from build123d import *

# Parameters (mm, degrees)
SKETCH1_W            = 39
SKETCH1_H            = 122
BOSS_EXTRUDE2_DEPTH  = 2
SKETCH2_W            = 2
SKETCH2_H            = 122
BOSS_EXTRUDE3_DEPTH  = 25
SKETCH3_W            = 2
SKETCH3_H            = 122
BOSS_EXTRUDE4_DEPTH  = 25
SKETCH4_W            = 35
SKETCH4_H            = 2
BOSS_EXTRUDE5_DEPTH  = 25
FILLET2_R            = 2
BOSS_EXTRUDE7_DEPTH  = 4
CUT_EXTRUDE2_DEPTH   = 4
SKETCH5_W            = 4
SKETCH5_H            = 9
CUT_EXTRUDE3_DEPTH   = 4
FILLET4_R            = 2
SKETCH8_W            = 7
SKETCH8_H            = 7
BOSS_EXTRUDE8_DEPTH  = 7
SKETCH9_W            = 7
SKETCH9_H            = 7
BOSS_EXTRUDE10_DEPTH = 7
SKETCH10_R           = 2
CUT_EXTRUDE6_DEPTH   = 7
SKETCH11_W           = 7
SKETCH11_H           = 7
BOSS_EXTRUDE11_DEPTH = 7
SKETCH12_R           = 2
CUT_EXTRUDE7_DEPTH   = 7


with BuildPart() as part:
    # Sketch1 → Boss-Extrude2 (new body)
    with BuildSketch(Plane.XY):
        with Locations((19.5, 61)):
            Rectangle(SKETCH1_W, SKETCH1_H)
    extrude(amount=BOSS_EXTRUDE2_DEPTH)

    # Sketch2 → Boss-Extrude3 (add)
    with BuildSketch(Plane(origin=(0, 0, 0), x_dir=(-1, 0, 0), z_dir=(0, 0, -1))):
        with Locations((-38, 61)):
            Rectangle(SKETCH2_W, SKETCH2_H)
    extrude(amount=BOSS_EXTRUDE3_DEPTH)

    # Sketch3 → Boss-Extrude4 (add)
    with BuildSketch(Plane(origin=(0, 0, 0), x_dir=(-1, 0, 0), z_dir=(0, 0, -1))):
        with Locations((-1, 61)):
            Rectangle(SKETCH3_W, SKETCH3_H)
    extrude(amount=BOSS_EXTRUDE4_DEPTH)

    # Sketch4 → Boss-Extrude5 (add)
    with BuildSketch(Plane(origin=(0, 0, 0), x_dir=(-1, 0, 0), z_dir=(0, 0, -1))):
        with Locations((-19.5, 1)):
            Rectangle(SKETCH4_W, SKETCH4_H)
    extrude(amount=BOSS_EXTRUDE5_DEPTH)

    # Fillet2
    fillet2_edges = [part.edges().sort_by_distance(p)[0] for p in [
        (19.5, 0, 2),
        (0, 0, -11.5),
        (39, 0, -11.5),
    ]]
    fillet(fillet2_edges, radius=FILLET2_R)

    # Sketch6 → Boss-Extrude7 (add)
    with BuildSketch(Plane(origin=(0, 0, -25), x_dir=(-1, 0, 0), z_dir=(0, 0, -1))):
        with BuildLine():
            Line((-2, 122), (0, 122))
            Line((0, 122), (0, 2))
            ThreePointArc((0, 2), (-0.585786438, 0.585786438), (-2, 0))
            Line((-2, 0), (-37, 0))
            ThreePointArc((-37, 0), (-38.414213562, 0.585786438), (-39, 2))
            Line((-39, 2), (-39, 122))
            Line((-39, 122), (-37, 122))
            Line((-37, 122), (-37, 2))
            Line((-37, 2), (-2, 2))
            Line((-2, 2), (-2, 122))
        make_face()
    extrude(amount=BOSS_EXTRUDE7_DEPTH)

    # Sketch7 → Cut-Extrude2 (cut)
    with BuildSketch(Plane.ZY):
        with BuildLine():
            Line((-21.5, 110), (-20.5, 110))
            ThreePointArc((-20.5, 110), (-19.439339828, 109.560660172), (-19, 108.5))
            Line((-19, 108.5), (-19, 102.5))
            ThreePointArc((-19, 102.5), (-19.439339828, 101.439339828), (-20.5, 101))
            Line((-20.5, 101), (-21.5, 101))
            ThreePointArc((-21.5, 101), (-22.560660172, 101.439339828), (-23, 102.5))
            Line((-23, 102.5), (-23, 108.5))
            ThreePointArc((-23, 108.5), (-22.560660172, 109.560660172), (-21.5, 110))
        make_face()
    extrude(amount=-CUT_EXTRUDE2_DEPTH, mode=Mode.SUBTRACT)

    # Sketch5 → Cut-Extrude3 (cut)
    with BuildSketch(Plane(origin=(39, 0, 0), x_dir=(0, 0, -1), z_dir=(1, 0, 0))):
        with Locations((21, 105.5)):
            Rectangle(SKETCH5_W, SKETCH5_H)
    extrude(amount=-CUT_EXTRUDE3_DEPTH, mode=Mode.SUBTRACT)

    # Fillet4
    # the kernel refuses this fillet: 2 mm, written as the material it takes off along each edge
    with BuildSketch(Plane(origin=(37, 2, 0), x_dir=(1, 0, 0), z_dir=(0, 0, 1))) as fillet4_piece_1_section:
        Polygon((0, 0), (FILLET4_R, 0), (FILLET4_R, -FILLET4_R), (0, -FILLET4_R), align=None)
    fillet4_piece_1 = extrude(amount=FILLET4_R, mode=Mode.PRIVATE)
    fillet4_piece_1 = fillet4_piece_1 - Plane(origin=(37, 2, 0), x_dir=(-0.7071067811865476, 0.7071067811865475, 0), z_dir=(0, 0, 1)) * Sphere(FILLET4_R, mode=Mode.PRIVATE)
    add(fillet4_piece_1, mode=Mode.SUBTRACT)
    with BuildSketch(Plane(origin=(2, 2, 0), x_dir=(0, 0, 1), z_dir=(-1, 0, 0))) as fillet4_piece_2_section:
        Polygon((0, 0), (FILLET4_R, 0), (FILLET4_R, -FILLET4_R), (0, -FILLET4_R), align=None)
    fillet4_piece_2 = extrude(amount=FILLET4_R, mode=Mode.PRIVATE)
    fillet4_piece_2 = fillet4_piece_2 - Plane(origin=(2, 2, 0), x_dir=(0, 0.7071067811865475, -0.7071067811865475), z_dir=(-1, 0, 0)) * Sphere(FILLET4_R, mode=Mode.PRIVATE)
    add(fillet4_piece_2, mode=Mode.SUBTRACT)
    with BuildSketch(Plane(origin=(0, 2, 2), x_dir=(0, 0, -1), z_dir=(0, 1, 0))) as fillet4_piece_3:
        with BuildLine():
            CenterArc((FILLET4_R, -FILLET4_R), FILLET4_R, 90, 90)
            Line((0, -FILLET4_R), (0, 0))
            Line((0, 0), (FILLET4_R, 0))
        make_face()
    extrude(amount=125, mode=Mode.SUBTRACT)
    with BuildSketch(Plane(origin=(39, 127, 2), x_dir=(-1, 0, 0), z_dir=(0, -1, 0))) as fillet4_piece_4:
        with BuildLine():
            CenterArc((FILLET4_R, FILLET4_R), FILLET4_R, 180, 90)
            Line((0, FILLET4_R), (0, 0))
            Line((0, 0), (FILLET4_R, 0))
        make_face()
    extrude(amount=125, mode=Mode.SUBTRACT)

    # Sketch8 → Boss-Extrude8 (add)
    with BuildSketch(Plane(origin=(0, 0, -29), x_dir=(-1, 0, 0), z_dir=(0, 0, -1))):
        with Locations((-33.5, 5.5)):
            Rectangle(SKETCH8_W, SKETCH8_H)
    extrude(amount=-BOSS_EXTRUDE8_DEPTH)

    # Sketch9 → Boss-Extrude10 (add)
    with BuildSketch(Plane(origin=(0, 0, -29), x_dir=(-1, 0, 0), z_dir=(0, 0, -1))):
        with Locations((-5.5, 5.5)):
            Rectangle(SKETCH9_W, SKETCH9_H)
    extrude(amount=-BOSS_EXTRUDE10_DEPTH)

    # Sketch10 → Cut-Extrude6 (cut)
    with BuildSketch(Plane(origin=(0, 0, -29), x_dir=(-1, 0, 0), z_dir=(0, 0, -1))):
        with Locations((-33.5, 5.5)):
            Circle(SKETCH10_R)
        with Locations((-5.5, 5.5)):
            Circle(SKETCH10_R)
    extrude(amount=-CUT_EXTRUDE6_DEPTH, mode=Mode.SUBTRACT)

    # Sketch11 → Boss-Extrude11 (add)
    with BuildSketch(Plane(origin=(0, 122, 0), x_dir=(1, 0, 0), z_dir=(0, 1, 0))):
        with Locations((5.5, 3.5)):
            Rectangle(SKETCH11_W, SKETCH11_H)
        with Locations((33.5, 3.5)):
            Rectangle(SKETCH11_W, SKETCH11_H)
        with Locations((5.5, 25.5)):
            Rectangle(SKETCH11_W, SKETCH11_H)
        with Locations((33.5, 25.5)):
            Rectangle(SKETCH11_W, SKETCH11_H)
    extrude(amount=-BOSS_EXTRUDE11_DEPTH)

    # Sketch12 → Cut-Extrude7 (cut)
    with BuildSketch(Plane(origin=(0, 122, 0), x_dir=(1, 0, 0), z_dir=(0, 1, 0))):
        with Locations(Location((5.5, 25.5, 0), (0, 0, 270))):
            Circle(SKETCH12_R)
        with Locations(Location((33.5, 25.5, 0), (0, 0, 270))):
            Circle(SKETCH12_R)
        with Locations(Location((5.5, 3.5, 0), (0, 0, 270))):
            Circle(SKETCH12_R)
        with Locations(Location((33.5, 3.5, 0), (0, 0, 270))):
            Circle(SKETCH12_R)
    extrude(amount=-CUT_EXTRUDE7_DEPTH, mode=Mode.SUBTRACT)


solid = part.part
Verification items for the finished model (mm, model axes). A direction names the side the tool comes from. Coordinates: 2 decimals unless noted, no trailing zeros. Write each loop counter-clockwise with the first axis right and the second up, starting at its lowest first coordinate (ties: lowest second). Pieces come first, ordered by that corner, then holes. Notation, with made-up numbers: (1.5, -30) -> (43.5, -30) arc R18 ccw to (43.5, -7) -> close; hole circle Ø3 at (37, 77). An arc over 180 degrees is marked (long way). One line per item, written item: value. Start each with the question number.
Q1. Go/stop test with a flat-tipped pin: P1, Ø4, axis at x = 12.5, z = -3.5, coming from the +Y side. Record where the tip stops, or that it passes through.
Q2. Cross-section at D-D on y = 5.5. Enter the section's corners in (x, z).
Q3. Access from +Z, -Z, +X, -X, +Y, -Y to the whole of each face (thin tool, end or side, straight path). Record for faces 5 (the flat face through (5, 119, -7)), 6 (the flat face through (34, 9, -26)), 7 (the flat face through (9, 119, -25)), 8 (the flat face through (1, 106, -19)).
Q4. Cross-section at C-C on x = 33.5. Enter the section's corners in (y, z).
Q5. Cross-section at A-A on z = -25.5. Enter the section's corners in (x, y), and give its area (3 significant figures).
Q6. Cross-section at B-B on z = -3.5. Enter the section's corners in (x, y), and give its area (3 significant figures).
Q7. Thickness scan on L1, parallel to X at y = 119.25, z = -3.5; L2, parallel to X at y = 5.5, z = -8.5; L3, parallel to X at y = 117, z = -25. Record the ranges inside material, lowest first. Write a range as from..to.
Q8. Mould release check, pull along X, two halves, no side actions. Record for faces 1 (the flat face through (39, 61, -14)), 2 (the flat face through (31.9, 115, -24)), 3 (the cylindrical face through (0.57, 61.16, 1.4)), 4 (the flat face through (30, 119, -25)): pulls with the +X half, pulls with the -X half, needs draft (parallel to the pull), parting line crosses it, or undercut.
Checked values:
1. P1: stops at y = 2
2. outline: (0, -29) -> (3.5, -29) -> (3.5, -22) -> (2, -22) -> (2, 0) -> (37, 0) -> (37, -22) -> (35.5, -22) -> (35.5, -29) -> (39, -29) -> (39, 0) arc R2 ccw to (37, 2) -> (2, 2) arc R2 ccw to (0, 0) -> close; (7.5, -29) -> (9, -29) -> (9, -22) -> (7.5, -22) -> close; (30, -29) -> (31.5, -29) -> (31.5, -22) -> (30, -22) -> close
3. face 5: +Y
3. face 6: -Z
3. face 7: -Z, +Y
3. face 8: +X, -X
4. outline: (0, -29) -> (3.5, -29) -> (3.5, -22) -> (2, -22) -> (2, 0) -> (115, 0) -> (115, -1.5) -> (122, -1.5) -> (122, 2) -> (2, 2) arc R2 ccw to (0, 0) -> close; (7.5, -29) -> (9, -29) -> (9, -22) -> (7.5, -22) -> close; (115, -29) -> (122, -29) -> (122, -27.5) -> (115, -27.5) -> close; (115, -23.5) -> (122, -23.5) -> (122, -22) -> (115, -22) -> close; (115, -7) -> (122, -7) -> (122, -5.5) -> (115, -5.5) -> close
5. outline: (0, 2) arc R2 ccw to (2, 0) -> (37, 0) arc R2 ccw to (39, 2) -> (39, 122) -> (35.5, 122) -> (35.5, 115) -> (37, 115) -> (37, 9) -> (30, 9) -> (30, 2) -> (9, 2) -> (9, 9) -> (2, 9) -> (2, 115) -> (3.5, 115) -> (3.5, 122) -> (0, 122) -> close; (7.5, 115) -> (9, 115) -> (9, 122) -> (7.5, 122) -> close; (30, 115) -> (31.5, 115) -> (31.5, 122) -> (30, 122) -> close; hole circle Ø4 at (5.5, 5.5); hole circle Ø4 at (33.5, 5.5)
5. area: 671 mm²
6. outline: (0, 2) arc R2 ccw to (2, 0) -> (37, 0) arc R2 ccw to (39, 2) -> (39, 122) -> (35.5, 122) -> (35.5, 115) -> (37, 115) -> (37, 2) -> (2, 2) -> (2, 115) -> (3.5, 115) -> (3.5, 122) -> (0, 122) -> close; (7.5, 115) -> (9, 115) -> (9, 122) -> (7.5, 122) -> close; (30, 115) -> (31.5, 115) -> (31.5, 122) -> (30, 122) -> close
6. area: 598 mm²
7. L1: x = 0..3.5, 7.5..9, 30..31.5, 35.5..39
7. L2: x = 0..2, 37..39
7. L3: x = 0..3.56, 7.44..9, 30..31.56, 35.44..39
8. face 1: pulls with the +X half
8. face 2: undercut
8. face 3: pulls with the -X half
8. face 4: undercut
